from build123d import *

# Parameters (mm, degrees)
SKETCH1_R               = 74
SKETCH1_R_2             = 71
BOSS_EXTRUDE1_DEPTH     = 15
SKETCH2_R               = 6.5
CUT_EXTRUDE1_DEPTH      = 73
CUT_EXTRUDE1_DEPTH_BACK = 75
SKETCH9_R               = 5.5
CUT_EXTRUDE6_DEPTH      = 75.0000001
BOSS_EXTRUDE2_START     = -6
SKETCH3_R               = 5
BOSS_EXTRUDE2_DEPTH     = 7
SKETCH4_W               = 10.783766206
SKETCH4_H               = 4.5
SKETCH4_W_2             = 12.537472389
BOSS_EXTRUDE3_DEPTH     = 15
SKETCH5_R               = 0.9
CUT_EXTRUDE2_DEPTH      = 8
SKETCH6_R               = 2.45
CUT_EXTRUDE3_DEPTH      = 4
SKETCH7_R               = 1.25
CUT_EXTRUDE4_DEPTH      = 4
SKETCH8_R               = 2.5
CUT_EXTRUDE5_DEPTH      = 4


with BuildPart() as part:
    # Sketch1 → Boss-Extrude1 (new body)
    with BuildSketch(Plane(origin=(0, 0, 0), x_dir=(1, 0, 0), z_dir=(0, 1, 0))):
        Circle(SKETCH1_R)
        Circle(SKETCH1_R_2, mode=Mode.SUBTRACT)
    extrude(amount=BOSS_EXTRUDE1_DEPTH)

    # Sketch2 → Cut-Extrude1 (cut, two sides)
    with BuildSketch(Plane(origin=(0, 0, 0), x_dir=(0, 0, -1), z_dir=(1, 0, 0))) as cut_extrude1_sk:
        with Locations((0, 7.5)):
            Circle(SKETCH2_R)
    extrude(amount=CUT_EXTRUDE1_DEPTH, mode=Mode.SUBTRACT)
    extrude(cut_extrude1_sk.sketch, amount=-CUT_EXTRUDE1_DEPTH_BACK, mode=Mode.SUBTRACT)

    # Sketch9 → Cut-Extrude6 (cut, through all)
    with BuildSketch(Plane(origin=(0, 0, 0), x_dir=(0, 0, -1), z_dir=(1, 0, 0))):
        with Locations((0, 7.5)):
            Circle(SKETCH9_R)
    extrude(amount=CUT_EXTRUDE6_DEPTH, mode=Mode.SUBTRACT)

    # Sketch3 → Boss-Extrude2 (add)
    with BuildSketch(Plane.XY.offset(73).offset(BOSS_EXTRUDE2_START)):
        with Locations((0, 7.5)):
            Circle(SKETCH3_R)
    boss_extrude2 = extrude(amount=BOSS_EXTRUDE2_DEPTH)

    # Mirror1: Boss-Extrude2 across plane
    add(boss_extrude2.mirror(Plane.XY))

    # Sketch4 → Boss-Extrude3 (add)
    with BuildSketch(Plane(origin=(0, 15, 0), x_dir=(1, 0, 0), z_dir=(0, 1, 0))):
        with Locations((-63.591883103, -19.05)):
            Rectangle(SKETCH4_W, SKETCH4_H)
        with Locations((-64.468736194, 8.35)):
            Rectangle(SKETCH4_W_2, SKETCH4_H)
    extrude(amount=-BOSS_EXTRUDE3_DEPTH)

    # Sketch5 → Cut-Extrude2 (cut)
    with BuildSketch(Plane(origin=(-58.2, 0, 0), x_dir=(0, 0, -1), z_dir=(1, 0, 0))):
        with Locations((8.3, 7.5)):
            Circle(SKETCH5_R)
        with Locations((-19, 7.5)):
            Circle(SKETCH5_R)
    extrude(amount=-CUT_EXTRUDE2_DEPTH, mode=Mode.SUBTRACT)

    # Sketch6 → Cut-Extrude3 (cut)
    with BuildSketch(Plane(origin=(0, 0, 67), x_dir=(-1, 0, 0), z_dir=(0, 0, -1))):
        with Locations((0, 7.5)):
            Circle(SKETCH6_R)
    extrude(amount=-CUT_EXTRUDE3_DEPTH, mode=Mode.SUBTRACT)

    # Sketch7 → Cut-Extrude4 (cut)
    with BuildSketch(Plane(origin=(0, 0, 71), x_dir=(-1, 0, 0), z_dir=(0, 0, -1))):
        with Locations((0, 7.5)):
            Circle(SKETCH7_R)
    extrude(amount=-CUT_EXTRUDE4_DEPTH, mode=Mode.SUBTRACT)

    # Sketch8 → Cut-Extrude5 (cut)
    with BuildSketch(Plane(origin=(0, 0, 73), x_dir=(-1, 0, 0), z_dir=(0, 0, -1))):
        with Locations((0, 7.5)):
            Circle(SKETCH8_R)
    extrude(amount=-CUT_EXTRUDE5_DEPTH, mode=Mode.SUBTRACT)


solid = part.part
The listing builds one solid part. Answer for the finished solid, in the listing's coordinates (mm). A direction names the side the tool comes from. Give positions to 0.01 mm unless a question says otherwise; leave off trailing zeros. Write each loop counter-clockwise with the first axis right and the second up, starting at its lowest first coordinate (ties: lowest second). Pieces come first, ordered by that corner, then holes. Notation, with made-up numbers: (-11, 0) -> (35, 0) arc R14 cw to (35, 23) -> close; hole circle Ø6 at (77.25, 40.25). An arc over 180 degrees is marked (long way). Use a Markdown table: item, result.
(1) Section C-C, the plane x = -63.5 is taken. Determine the outline of the cut face in (y, z), then the cut area to 3 significant figures.
Return value:
| item | result |
|---|---|
| outline | (0, -38) -> (15, -38) -> (15, -31.76) -> (0, -31.76) -> close; (0, -10.6) -> (15, -10.6) -> (15, -6.1) -> (0, -6.1) -> close; (0, 16.8) -> (15, 16.8) -> (15, 21.3) -> (0, 21.3) -> close; (0, 31.76) -> (15, 31.76) -> (15, 38) -> (0, 38) -> close; hole circle Ø1.8 at (7.5, -8.3); hole circle Ø1.8 at (7.5, 19) |
| area | 317 mm2 |
(2) Section A-A, the plane x = 16 is taken. Determine the outline of the cut face in (y, z), then the cut area to 3 significant figures.
Return value:
| item | result |
|---|---|
| outline | (0, -72.25) -> (15, -72.25) -> (15, -69.17) -> (0, -69.17) -> close; (0, 69.17) -> (15, 69.17) -> (15, 72.25) -> (0, 72.25) -> close |
| area | 92.3 mm2 |
(3) Flat-ended cylindrical pins translate along their axes: P1, Ø5, axis at y = 6.5, z = 20, coming from the +X side; P2, Ø5, axis at x = -64.5, y = 9, coming from the +Z side; P3, Ø1.4, axis at y = 8, z = 19, coming from the +X side. Find the tip coordinate at first contact, or state that the pin passes through.
Return value:
| item | result |
|---|---|
| P1 | x = 71.9 |
| P2 | z = 40.4 |
| P3 | x = 71.7 |
(4) Find the intervals of material crossed by probe 1 along Y at (x, z) = (-72.2, 0); probe 2 along Z at (x, y) = (-1, 1.25); probe 3 along Z at (x, y) = (-59, 3.25), in increasing order. Write a range as from..to.
Return value:
| item | result |
|---|---|
| probe 1 | 0..1, 14..15 |
| probe 2 | -73.99..-70.99, 70.99..73.99 |
| probe 3 | -44.67..-39.5, -10.6..-6.1, 16.8..21.3, 39.5..44.67 |
(5) Determine the mould class of faces 1 (the flat face through (-58.2, 8, 20)), 2 (the cylindrical face through (-0.651, 12.457, -68.972)), 3 (the cylindrical face through (71.835, 1.155, 1.409)), 4 (the cylindrical face through (0.54, 5.06, 73.49)) for opening direction Y: released by +Y, released by -Y, zero draft, split by the parting line, or undercut.
Return value:
| item | result |
|---|---|
| face 1 | zero draft |
| face 2 | split by the parting line |
| face 3 | undercut |
| face 4 | undercut |
(6) For faces 5 (the cylindrical face through (0.5, 5.1, 69)), 6 (the flat face through (-1, 5, 67)), 7 (the flat face through (-66, 15, -28)), determine the directions among +Z, -Z, +X, -X, +Y, -Y from which every point of the face is accessible in a straight line to the end or side of a thin tool.
Return value:
| item | result |
|---|---|
| face 5 | none |
| face 6 | +Y, -Y |
| face 7 | +Z, -Z, +X, -X, +Y |
(7) Section B-B, the plane z = 57.5 is taken. Determine the outline of the cut face in (x, y), then the cut area to 3 significant figures.
Return value:
| item | result |
|---|---|
| outline | (-46.58, 0) -> (-41.65, 0) -> (-41.65, 15) -> (-46.58, 15) -> close; (41.65, 0) -> (46.58, 0) -> (46.58, 15) -> (41.65, 15) -> close |
| area | 148 mm2 |
